from build123d import *

# Parameters (mm, degrees)
ESQUISSE1_R        = 1.5
BOSS_EXTRU_1_DEPTH = 5


with BuildPart() as part:
    # Esquisse1 → Boss.-Extru.1 (new body)
    with BuildSketch(Plane.XY):
        with BuildLine():
            Line((0, 8), (20, 8))
            Line((20, 8), (20, -8))
            Line((20, -8), (0, -8))
            ThreePointArc((0, -8), (-8, 0), (0, 8))
        make_face()
        Circle(ESQUISSE1_R, mode=Mode.SUBTRACT)
        with Locations((15, 0)):
            Circle(ESQUISSE1_R, mode=Mode.SUBTRACT)
    extrude(amount=BOSS_EXTRU_1_DEPTH)


solid = part.part
Check sheet for the modelled part. Datum: model origin and axes. Units: mm. Give positions to 0.01 mm unless a question says otherwise; leave off trailing zeros. Loops run counter-clockwise (first coordinate to the right, second up) from the corner with the lowest first, then second, coordinate; pieces in that order, holes last. Notation, with made-up numbers: M -27.75,52 L 0.25,52 A27 cw 0.25,70 Z; hole C 56.5,-29 d7. An arc over 180 degrees is marked long. Answer as a JSON object with one key per item and string values. Group by question number.
Q1. Material ranges on line 1 along Y through (x, z) = (0, 3.65); line 2 along X through (y, z) = (0.25, 4.55); line 3 along Y through (x, z) = (-1.25, 1.25), recorded low to high. Write a range as [from, to].
Q2. Cross-section at D-D on x = -5.5. Record the cut outline in (y, z).
Q3. Cross-section at A-A on y = 0. Record the cut outline in (x, z).
Q4. Cross-section at C-C on z = 2.05. Record the cut outline in (x, y), then the cut area to 3 significant figures.
Q5. Release check for a two-part mould opening along Y. For faces 1 (the cylindrical face through (-8, 0, 2)), 2 (the cylindrical face through (13.5, 0.07, 2.46)), 3 (the cylindrical face through (-1.5, 0.07, 2.46)), 4 (the flat face through (20, 0, 2)) record: released by +Y, released by -Y, zero draft, split by the parting line, or undercut.
Q6. Go/stop test with flat-tipped pins: P1, Ø1.5, axis at x = 13.5, y = -5.5, coming from the -Z side; P2, Ø1, axis at x = -5, z = 2, coming from the +Y side; P3, Ø3, axis at y = 4.5, z = 1, coming from the -X side. Record where each tip stops, or that it passes through.
Q7. Cross-section at B-B on x = 15. Record the cut outline in (y, z).
Evaluation:
{
 "1": {"line 1": "y = [-8, -1.5], [1.5, 8]", "line 2": "x = [-8, -1.48], [1.48, 13.52], [16.48, 20]", "line 3": "y = [-7.9, -0.83], [0.83, 7.9]"},
 "2": {"outline": "M -5.81,0 L 5.81,0 L 5.81,5 L -5.81,5 Z"},
 "3": {"outline": "M -8,0 L -1.5,0 L -1.5,5 L -8,5 Z; M 1.5,0 L 13.5,0 L 13.5,5 L 1.5,5 Z; M 16.5,0 L 20,0 L 20,5 L 16.5,5 Z"},
 "4": {"outline": "M 0,-8 L 20,-8 L 20,8 L 0,8 A8 ccw Z; hole C 0,0 d3; hole C 15,0 d3", "area": "406 mm2"},
 "5": {"face 1": "split by the parting line", "face 2": "undercut", "face 3": "undercut", "face 4": "zero draft"},
 "6": {"P1": "stops at z = 0", "P2": "stops at y = 6.61", "P3": "stops at x = -7.42"},
 "7": {"outline": "M -8,0 L -1.5,0 L -1.5,5 L -8,5 Z; M 1.5,0 L 8,0 L 8,5 L 1.5,5 Z"}
}
